Design review of the part shown in the three views and the two pictorial views. Dimensions are in mm from the part's minimum x, y and z. A direction names the side the tool comes from. Coordinates: 2 decimals unless noted, no trailing zeros. Loops run counter-clockwise (first coordinate to the right, second up) from the corner with the lowest first, then second, coordinate; pieces in that order, holes last. Notation, with made-up numbers: (72, 45.5) -> (113, 45.5) arc R26 ccw to (113, 63.5) -> close; hole circle Ø5 at (-21.5, 34). An arc over 180 degrees is marked (long way). One line per item, written item: value. Start each with the question number.
1. Add section A-A on y = 23. Write out the cut boundary in (x, z), plus the area to 3 significant figures.
2. For probe 1 along X at (y, z) = (21.5, 7.75); probe 2 along Y at (x, z) = (10, 9); probe 3 along Y at (x, z) = (7.25, 10.5), list the stretches that pass through material, from the lowest coordinate up.
3. Machinability: for the marked faces 1 and 2, which of the approach directions +Z, -Z, +X, -X, +Y, -Y give a long, thin tool a straight path to every point of the face, cutting with its end or side? Answer none if there is none.
4. Add section C-C on x = 7. Write out the cut boundary in (y, z), plus the area to 3 significant figures.
5. Add section B-B on z = 8.85. Write out the cut boundary in (x, y).
6. Add section D-D on x = 10. Write out the cut boundary in (y, z), plus the area to 3 significant figures.
7. Draft analysis for pull direction X (two halves, no side actions). For the marked faces 3, 4, 5 and 6, state which applies: pulls with the +X half, pulls with the -X half, needs draft (parallel to the pull), parting line crosses it, or undercut.
8. Insertion check: pin 1 (10 mm diameter, centred on y = 8.85, z = 8.85, fed in from -X); pin 2 (4 mm diameter, centred on x = 5.5, z = 13, fed in from +Y). Each pin has a flat end and moves straight along its axis. Give the tip position at first contact, or say it passes through.
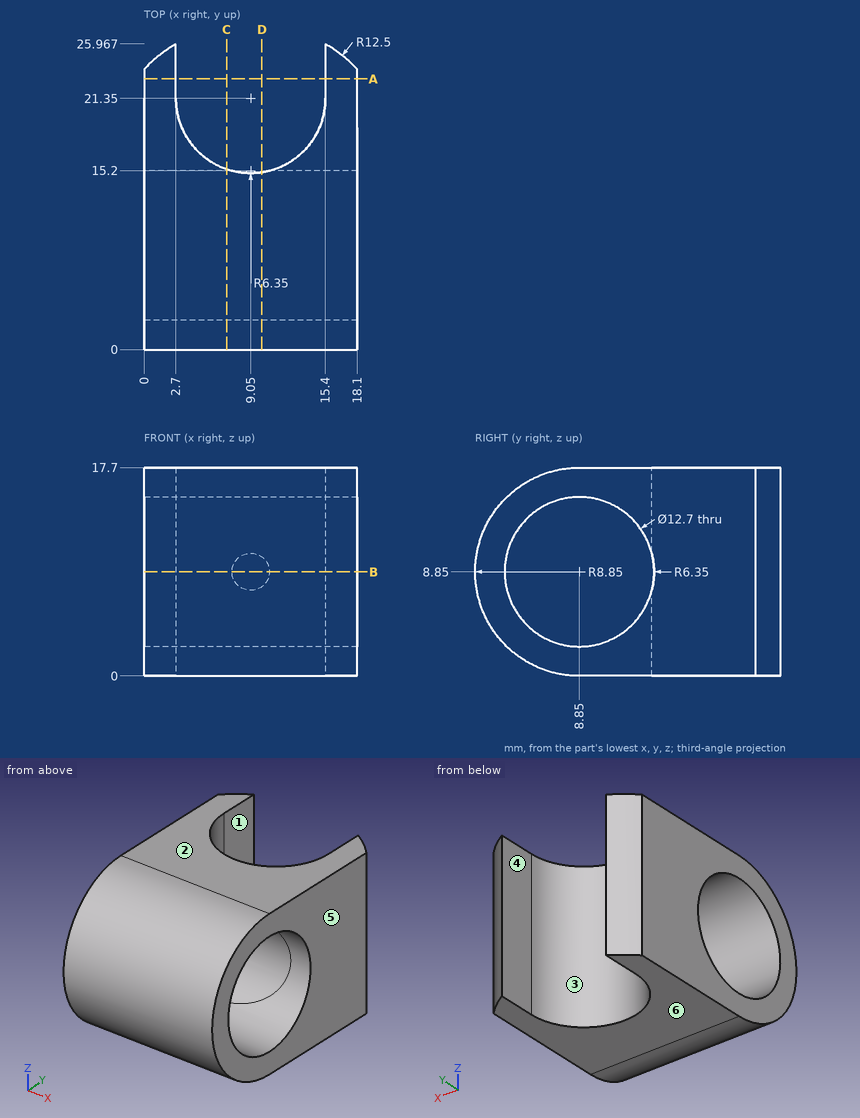
Worked answers:
1. outline: (0, 0) -> (2.7, 0) -> (2.7, 17.7) -> (0, 17.7) -> close; (15.4, 0) -> (18.1, 0) -> (18.1, 17.7) -> (15.4, 17.7) -> close
1. area: 95.6 mm²
2. probe 1: x = 0 to 2.7, 15.4 to 18.1
2. probe 2: y = 0 to 2.5
2. probe 3: y = 0.16 to 2.72, 14.98 to 15.26
3. face 1: +Z, -Z, +Y
3. face 2: +Z, +X, -X, +Y, -Y
4. outline: (8.85, 0) -> (15.34, 0) -> (15.34, 17.7) -> (8.85, 17.7) arc R8.85 ccw to start; hole circle Ø12.7 at (8.85, 8.85)
4. area: 111 mm²
5. outline: (0, 0) -> (18.1, 0) -> (18.1, 2.5) -> (0, 2.5) -> close; (0, 15.2) -> (7.47, 15.2) arc R6.35 cw to (2.7, 21.35) -> (2.7, 25.97) arc R12.5 ccw to (0, 23.82) -> close; (10.63, 15.2) -> (18.1, 15.2) -> (18.1, 23.82) arc R12.5 ccw to (15.4, 25.97) -> (15.4, 21.35) arc R6.35 cw to start
6. outline: (8.85, 0) -> (15.07, 0) -> (15.07, 7.58) arc R6.35 cw (long way) to (15.07, 10.12) -> (15.07, 17.7) -> (8.85, 17.7) arc R8.85 ccw to start
6. area: 107 mm²
7. face 3: undercut
7. face 4: undercut
7. face 5: pulls with the +X half
7. face 6: needs draft
8. pin 1: passes through
8. pin 2: stops at y = 18.26
